```python
from build123d import *

# Parameters (mm, degrees)
F0_W     = 127
F0_H     = 22.225
F0_R     = 6.2865
F0_R_2   = 5
F1_DEPTH = 101.6
F2_R     = 6.35
F3_R     = 1.75
F4_DEPTH = 101.601


with BuildPart() as f1:
    # F0 (on Front) → F1 (new body)
    with BuildSketch(Plane.XZ):
        Rectangle(F0_W, F0_H)
        with Locations((-44.45, 0)):
            Circle(F0_R, mode=Mode.SUBTRACT)
        Circle(F0_R_2, mode=Mode.SUBTRACT)
        with Locations((44.45, 0)):
            Circle(F0_R, mode=Mode.SUBTRACT)
    extrude(amount=F1_DEPTH)

    # F2
    f2_edges = [f1.edges().sort_by_distance(p)[0] for p in [
        (-63.5, -50.8, -11.1125),
        (63.5, -50.8, -11.1125),
    ]]
    fillet(f2_edges, radius=F2_R)

    # F3 (on face) → F4 (cut, through all)
    with BuildSketch(Plane.XZ.offset(101.6)):
        with Locations((-5.656854, 5.656854)):
            Circle(F3_R)
        with Locations((5.656854, 5.656854)):
            Circle(F3_R)
        with Locations((5.656854, -5.656854)):
            Circle(F3_R)
        with Locations((-5.656854, -5.656854)):
            Circle(F3_R)
    extrude(amount=-F4_DEPTH, mode=Mode.SUBTRACT)


solid = f1.part
```
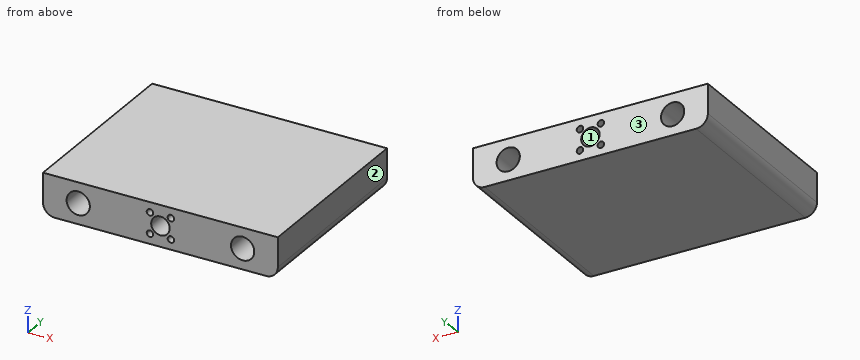
Can you work these out from the model? Positions are in its coordinate system, mm. Face numbers are marked on the shaded views. Coordinates: 2 decimals unless noted, no trailing zeros. Write each loop counter-clockwise with the first axis right and the second up, starting at its lowest first coordinate (ties: lowest second). Pieces come first, ordered by that corner, then holes. Notation, with made-up numbers: M 49,27.25 L 108,27.25 A25 ccw 108,49.25 Z; hole C 86,31 d7. An arc over 180 degrees is marked long. Write item = value, one per line. Start each with the question number.
Q1. If we section it at A-A, the plane x = 0: Write out the boundary of the cut face in (y, z), then the cut area to 3 significant figures.
Q2. If we section it at B-B, the plane z = 0: Write out the boundary of the cut face in (x, y), then the cut area to 3 significant figures.
Q3. Thinking about a two-plate mould opening in X: for the marked faces 1, 2 and 3, which applies, released by +X, released by -X, zero draft, split by the parting line, or undercut?
Q4. If we section it at C-C, the plane y = -60.5: Write out the boundary of the cut face in (x, z), then the cut area to 3 significant figures.
Q5. I'm going to push flat-ended pins straight in: pin 1 (5.5 mm diameter, centred on x = 5.66, z = -5.66, fed in from +Y); pin 2 (4 mm diameter, centred on y = -66, z = -7, fed in from +X); pin 3 (2 mm diameter, centred on x = 5.66, z = 5.66, fed in from +Y). Where does each tip first touch, or does it pass through?
Q6. If I drill on L1, parallel to Z at x = 44, y = -79; L2, parallel to X at y = -30.5, z = 1.75; L3, parallel to X at y = -86, z = -1.5, over which ranges is the centre line in solid material (lowest first)? Write a range as [from, to].
Q7. If we section it at D-D, the plane x = 44.45: Write out the boundary of the cut face in (y, z), then the cut area to 3 significant figures.
Check sheet entries:
q1.outline = M -101.6,-11.11 L 0,-11.11 L 0,-5 L -101.6,-5 Z; M -101.6,5 L 0,5 L 0,11.11 L -101.6,11.11 Z
q1.area = 1,240 mm²
q2.outline = M -63.5,-101.6 L -50.74,-101.6 L -50.74,0 L -63.5,0 Z; M -38.16,-101.6 L -5,-101.6 L -5,0 L -38.16,0 Z; M 5,-101.6 L 38.16,-101.6 L 38.16,0 L 5,0 Z; M 50.74,-101.6 L 63.5,-101.6 L 63.5,0 L 50.74,0 Z
q2.area = 9,330 mm²
q3.face_1 = undercut
q3.face_2 = released by +X
q3.face_3 = zero draft
q4.outline = M -63.5,-4.76 A6.35 ccw -57.15,-11.11 L 57.15,-11.11 A6.35 ccw 63.5,-4.76 L 63.5,11.11 L -63.5,11.11 Z; hole C -44.45,0 d12.57; hole C -5.66,-5.66 d3.5; hole C -5.66,5.66 d3.5; hole C 0,0 d10; hole C 5.66,-5.66 d3.5; hole C 5.66,5.66 d3.5; hole C 44.45,0 d12.57
q4.area = 2,440 mm²
q5.pin_1 = 0
q5.pin_2 = 63.5
q5.pin_3 = through
q6.L1 = [-11.11, -6.27], [6.27, 11.11]
q6.L2 = [-63.5, -50.49], [-38.41, -4.68], [4.68, 38.41], [50.49, 63.5]
q6.L3 = [-63.5, -50.55], [-38.35, -4.77], [4.77, 38.35], [50.55, 63.5]
q7.outline = M -101.6,-11.11 L 0,-11.11 L 0,-6.29 L -101.6,-6.29 Z; M -101.6,6.29 L 0,6.29 L 0,11.11 L -101.6,11.11 Z
q7.area = 981 mm²
